from build123d import *

# Parameters (mm, degrees)
MODEL_R                 = 1.7
MODEL_R_2               = 1.600279216
SALIENTE_EXTRUIR1_DEPTH = 3


with BuildPart() as part:
    # Model → Saliente-Extruir1 (new body)
    with BuildSketch(Plane.XY):
        with BuildLine():
            Line((60.263543448, -46.554934941), (60.263543448, -115.557339175))
            ThreePointArc((60.263543448, -115.557339175), (60.702883276, -116.617999347), (61.763543448, -117.057339175))
            Line((61.763543448, -117.057339175), (139.768153306, -117.057339175))
            ThreePointArc((139.768153306, -117.057339175), (140.828813478, -116.617999347), (141.268153306, -115.557339175))
            Line((141.268153306, -115.557339175), (141.268153306, -46.554934941))
            ThreePointArc((141.268153306, -46.554934941), (140.828813478, -45.494274769), (139.768153306, -45.054934941))
            Line((139.768153306, -45.054934941), (61.763543448, -45.054934941))
            ThreePointArc((61.763543448, -45.054934941), (60.702883276, -45.494274769), (60.263543448, -46.554934941))
        make_face()
        with Locations((136.768487808, -103.558008179)):
            Circle(MODEL_R, mode=Mode.SUBTRACT)
        with Locations((136.768487808, -58.554600438)):
            Circle(MODEL_R, mode=Mode.SUBTRACT)
        with Locations((136.768487808, -112.557673677)):
            Circle(MODEL_R_2, mode=Mode.SUBTRACT)
        with Locations((136.768487808, -49.554934941)):
            Circle(MODEL_R_2, mode=Mode.SUBTRACT)
        with Locations((64.763543448, -103.558008179)):
            Circle(MODEL_R, mode=Mode.SUBTRACT)
        with Locations((64.763543448, -58.554600438)):
            Circle(MODEL_R, mode=Mode.SUBTRACT)
        with Locations((64.763543448, -49.554934941)):
            Circle(MODEL_R_2, mode=Mode.SUBTRACT)
        with Locations((64.763543448, -112.557673677)):
            Circle(MODEL_R_2, mode=Mode.SUBTRACT)
        Polygon((71.651345037, -46.935116153), (131.055954895, -46.935116153), (132.855954895, -48.735116152), (132.855954895, -60.048667687), (134.855954895, -61.435116153), (138.055954895, -61.435116153), (138.855954895, -62.235116152), (138.855954895, -99.637520387), (138.055954895, -100.437520387), (134.855954895, -100.437520387), (132.855954895, -102.421405318), (132.855954895, -114.137520387), (132.055954895, -114.937520387), (69.451345037, -114.937520387), (68.651345037, -114.137520387), (68.651345037, -101.317509753), (67.851345037, -100.437520387), (64.651345037, -100.437520387), (62.851345037, -98.637520387), (62.851345037, -63.235116152), (64.651345037, -61.435116153), (67.851345037, -61.435116153), (69.851345037, -58.49810879), (69.851345037, -48.735116152), align=None, mode=Mode.SUBTRACT)
    extrude(amount=SALIENTE_EXTRUIR1_DEPTH)


solid = part.part
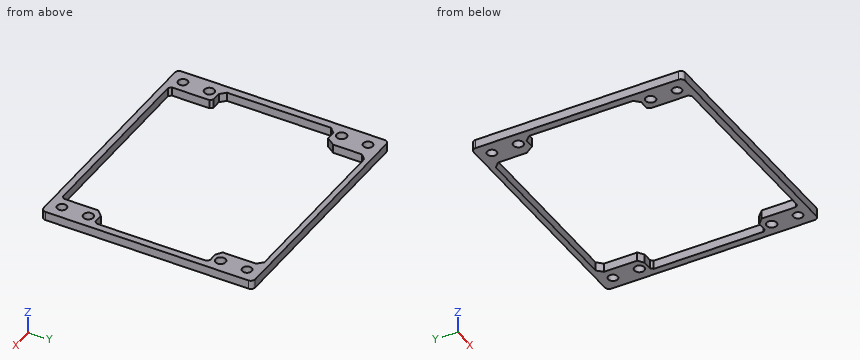
Part model, mm, in its own coordinate system. Coordinates: 2 decimals unless noted, no trailing zeros. Order: outer loops, then holes, each group sorted by start corner. A loop starts at its lowest first (then second) coordinate and runs counter-clockwise, first axis right, second up. Notation, with made-up numbers: M -14,-10.75 L 31,-10.75 A20 cw 31,13.25 Z; hole C -7,-37 d1. An arc over 180 degrees is marked long. One line per question, with ' | ' between items.
Q1. Drill centre lines: line 1 (X direction, y = -112.5, z = 1.4); line 2 (Y direction, x = 137, z = 0.9); line 3 (Y direction, x = 128.5, z = 2.3). Where is each one in solid material? Low to high.
A:
line 1: x = 60.26 to 63.16, 66.36 to 68.65, 132.86 to 135.17, 138.37 to 141.27 | line 2: y = -117.06 to -114.14, -110.97 to -105.24, -101.87 to -100.44, -61.44 to -60.24, -56.87 to -51.14, -47.97 to -45.05 | line 3: y = -117.06 to -114.94, -46.94 to -45.05
Q2. Slice it at B-B (y = -96.5). Give the cut face in (x, z).
A:
outline: M 60.26,0 L 62.85,0 L 62.85,3 L 60.26,3 Z; M 138.86,0 L 141.27,0 L 141.27,3 L 138.86,3 Z
Q3. Slice it at C-C (z = 2.4). Count the separate pieces of the cut face and the enclosed holes in it, and give its area (3 significant figures).
A:
separate pieces: 1 | enclosed holes: 9 | area: 954 mm^2
Q4. Slice it at A-A (x = 97.5). Give the cut face in (y, z), and give its area (3 significant figures).
A:
outline: M -117.06,0 L -114.94,0 L -114.94,3 L -117.06,3 Z; M -46.94,0 L -45.05,0 L -45.05,3 L -46.94,3 Z | area: 12.0 mm^2
Q5. Pin check, flat tip, straight feed: P1, Ø3, axis at x = 64.76, y = -112.56, coming from the -Z side. Stop position of the tip, or through.
A:
P1: passes through
